Can you work these out from the model? Positions are in its coordinate system, mm. Give positions to 0.01 mm unless a question says otherwise; leave off trailing zeros. Order: outer loops, then holes, each group sorted by start corner. A loop starts at its lowest first (then second) coordinate and runs counter-clockwise, first axis right, second up. Notation, with made-up numbers: M 58,16 L 86,16 A19 cw 86,29 Z; hole C 65,45.25 d9. An arc over 180 degrees is marked long. Use one line per item in the form item = value. Start each with the question number.
1. I need wall thicknesses on L1, parallel to X at y = 1.8, z = 67; L2, parallel to Z at x = 11, y = 1.9; L3, parallel to Z at x = 14.5, y = 2.7. Which ranges of each line are inside material? Lowest first, please.
2. I want a section at D-D, the plane x = -18.5. List the corners of the cut face in (y, z) for me, and give its area (3 significant figures).
3. I want a section at A-A, the plane x = -3.5. List the corners of the cut face in (y, z) for me.
4. I want a section at C-C, the plane x = 23.5. List the corners of the cut face in (y, z) for me, and give its area (3 significant figures).
5. I want a section at B-B, the plane y = 2.2. Count the separate pieces of the cut face and the enclosed holes in it, and give its area (3 significant figures).
6. Will these pins go through, and if not, where does the flat tip stop? P1, Ø1.4, axis at x = 39.5, y = 2, coming from the +Z side; P2, Ø1.4, axis at y = 1, z = 68, coming from the -X side; P3, Ø1.4, axis at y = 1.5, z = -22.5, coming from the -X side.
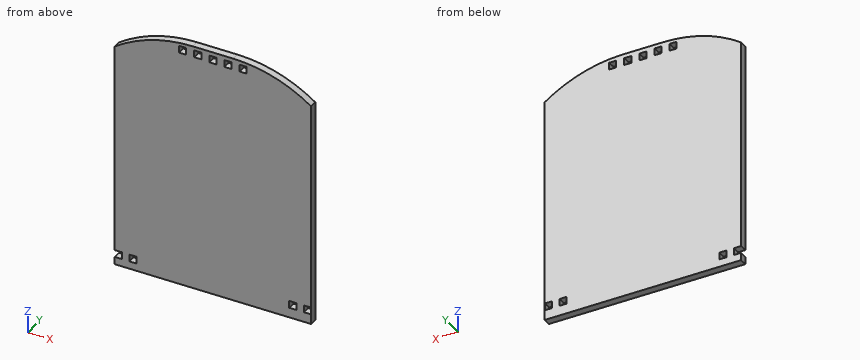
```python
from build123d import *

# Parameters (mm, degrees)
SKETCH1_W           = 2.8
SKETCH1_H           = 2.8
BOSS_EXTRUDE1_DEPTH = 3


with BuildPart() as part:
    # Sketch1 → Boss-Extrude1 (new body)
    with BuildSketch(Plane(origin=(0, 0, 0), x_dir=(1, 0, 0), z_dir=(0, 1, 0))):
        with BuildLine():
            Line((-36.479854722, 28.001428065), (-36.479854722, 25.001428065))
            Line((-36.479854722, 25.001428065), (-33.679854722, 25.001428065))
            Line((-33.679854722, 25.001428065), (-33.679854722, 22.201428065))
            Line((-33.679854722, 22.201428065), (-36.479854722, 22.201428065))
            Line((-36.479854722, 22.201428065), (-36.479854722, -61.498571935))
            ThreePointArc((-36.479854722, -61.498571935), (-21.743078282, -68.818947396), (-5.482204259, -71.337767111))
            Line((-5.482204259, -71.337767111), (10.522494814, -71.337767111))
            ThreePointArc((10.522494814, -71.337767111), (26.783368837, -68.818947396), (41.520145278, -61.498571935))
            Line((41.520145278, -61.498571935), (41.520145278, 28.001428065))
            Line((41.520145278, 28.001428065), (-36.479854722, 28.001428065))
        make_face()
        with Locations((-29.279854722, 23.601428065)):
            Rectangle(SKETCH1_W, SKETCH1_H, mode=Mode.SUBTRACT)
        with Locations((-9.479854722, -68.437767111)):
            Rectangle(SKETCH1_W, SKETCH1_H, mode=Mode.SUBTRACT)
        with Locations((-3.479854722, -68.437767111)):
            Rectangle(SKETCH1_W, SKETCH1_H, mode=Mode.SUBTRACT)
        with Locations((2.520145278, -68.237767111)):
            Rectangle(SKETCH1_W, SKETCH1_H, mode=Mode.SUBTRACT)
        with Locations((8.520145278, -68.237767111)):
            Rectangle(SKETCH1_W, SKETCH1_H, mode=Mode.SUBTRACT)
        with Locations((14.520145278, -68.237767111)):
            Rectangle(SKETCH1_W, SKETCH1_H, mode=Mode.SUBTRACT)
        with Locations((34.252496444, 22.650704456)):
            Rectangle(SKETCH1_W, SKETCH1_H, mode=Mode.SUBTRACT)
        with Locations((40.052496444, 22.650704456)):
            Rectangle(SKETCH1_W, SKETCH1_H, mode=Mode.SUBTRACT)
    extrude(amount=BOSS_EXTRUDE1_DEPTH)


solid = part.part
```
Check result:
q1.L1 = -26.64 to 1.12, 3.92 to 7.12, 9.92 to 13.12, 15.92 to 31.68
q1.L2 = -28 to 71.34
q1.L3 = -28 to 66.84, 69.64 to 71.19
q2.outline = M 0,-28 L 3,-28 L 3,69.74 L 0,69.74 Z
q2.area = 293 mm2
q3.outline = M 0,-28 L 3,-28 L 3,67.04 L 0,67.04 Z; M 0,69.84 L 3,69.84 L 3,71.34 L 0,71.34 Z
q4.outline = M 0,-28 L 3,-28 L 3,69.75 L 0,69.75 Z
q4.area = 293 mm2
q5.separate_pieces = 1
q5.enclosed_holes = 8
q5.area = 7,480 mm2
q6.P1 = 63.3
q6.P2 = -25.92
q6.P3 = -36.48
